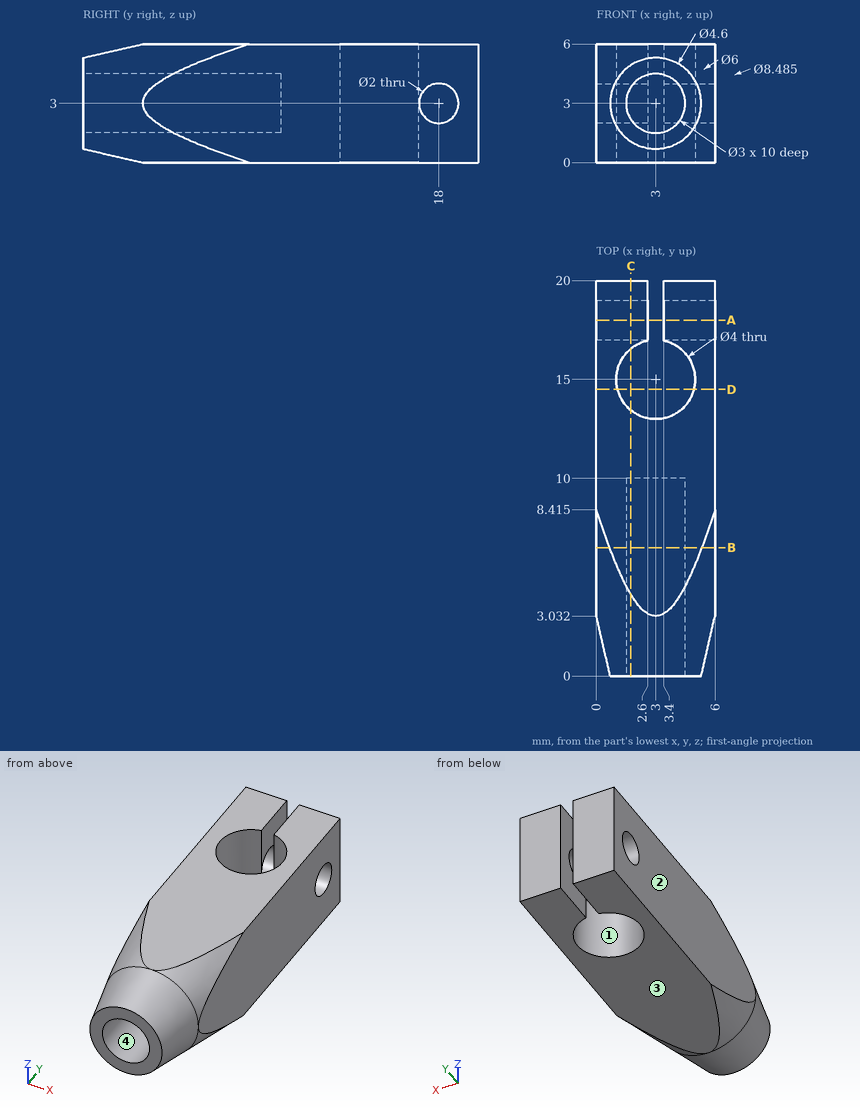
Drawing for the job (mm, zero at the part's lowest x, y, z). Round coordinates to 2 decimals unless told otherwise and drop trailing zeros. Write each loop counter-clockwise with the first axis right and the second up, starting at its lowest first coordinate (ties: lowest second). Pieces come first, ordered by that corner, then holes. Notation, with made-up numbers: M 2,61 L 46,61 A5 cw 46,66 Z; hole C 86.5,-12.5 d6. An arc over 180 degrees is marked long. Put each result on its own line as item: value.
Item 1: Probe L1, parallel to Z at x = 3, y = 5.75; L2, parallel to X at y = 15, z = 3.75; L3, parallel to Y at x = 4.65, z = 3. List the from-to ranges inside material, lowest first. Write a range as from..to.
Responses:
L1: 0..1.5, 4.5..6
L2: 0..1, 5..6
L3: 0..13.87, 16.13..17, 19..20
Item 2: Cut at D-D (y = 14.5). List the corners of the cut face in (x, z).
Responses:
outline: M 0,0 L 1.06,0 L 1.06,6 L 0,6 Z; M 4.94,0 L 6,0 L 6,6 L 4.94,6 Z
Item 3: Cut at B-B (y = 6.5). List the corners of the cut face in (x, z), and give its area (3 significant figures).
Responses:
outline: M 0,0.67 A3.8 ccw 0.67,0 L 5.33,0 A3.8 ccw 6,0.67 L 6,5.33 A3.8 ccw 5.33,6 L 0.67,6 A3.8 ccw 0,5.33 Z; hole C 3,3 d3
area: 28.1 mm²
Item 4: Mould opens along X. For the marked faces 1, 2, 3 and 4 say: +X half, -X half, draft (parallel to the pull), parting line (faces both ways), or undercut.
Responses:
face 1: undercut
face 2: -X half
face 3: draft
face 4: undercut
Item 5: Cut at A-A (y = 18). List the corners of the cut face in (x, z), and give its area (3 significant figures).
Responses:
outline: M 0,0 L 2.6,0 L 2.6,2 L 0,2 Z; M 0,4 L 2.6,4 L 2.6,6 L 0,6 Z; M 3.4,0 L 6,0 L 6,2 L 3.4,2 Z; M 3.4,4 L 6,4 L 6,6 L 3.4,6 Z
area: 20.8 mm²
Item 6: Cut at C-C (x = 1.75). State how many separate pieces and enclosed holes the cut face has.
Responses:
separate pieces: 2
enclosed holes: 1
Item 7: Flat gauge pins, fed straight in: P1, Ø1.2, axis at y = 18, z = 3, coming from the -X side; P2, Ø0.9, axis at x = 2.5, z = 3, coming from the -Y side. Where does each tip first touch, or does it go through?
Responses:
P1: through
P2: y = 10
